from build123d import *

# Parameters (mm, degrees)
BOSS_EXTRUDE1_DEPTH = 0.43
SKETCH2_R           = 8.35
BOSS_EXTRUDE2_DEPTH = 1.7
CIRPATTERN1_COUNT   = 4
SKETCH3_R           = 7.25
BOSS_EXTRUDE3_DEPTH = 1.1
BOSS_EXTRUDE4_DEPTH = 3
FILLET1_R           = 0.4
FILLET2_R           = 1.5
FILLET3_R           = 6


with BuildPart() as part:
    # Sketch1 → Boss-Extrude1 (new body, symmetric)
    with BuildSketch(Plane.XY):
        Polygon((0, 0), (84.5, 0), (84.5, 6.75), (68.25, 6.75), (66.5, 4.25), (64.75, 6.75), (21.5, 6.75), (12.5, 4.5), (0, 4.5), align=None)
    boss_extrude1 = extrude(amount=BOSS_EXTRUDE1_DEPTH, both=True)

    # Sketch2 → Boss-Extrude2 (add)
    with BuildSketch(Plane.ZY):
        Circle(SKETCH2_R)
    extrude(amount=-BOSS_EXTRUDE2_DEPTH)

    # CirPattern1: Boss-Extrude1 ×4 about axis
    cirpattern1_axis = Axis((0, 0, 0), (1, 0, 0))
    for i in range(1, CIRPATTERN1_COUNT):
        add(boss_extrude1.rotate(cirpattern1_axis, i * 360 / CIRPATTERN1_COUNT))

    # Sketch3 → Boss-Extrude3 (add)
    with BuildSketch(Plane(origin=(84.5, 0, 0), x_dir=(0, 0, -1), z_dir=(1, 0, 0))):
        Circle(SKETCH3_R)
    extrude(amount=-BOSS_EXTRUDE3_DEPTH)

    # Sketch4 → Boss-Extrude4 (add)
    with BuildSketch(Plane(origin=(84.5, 0, 0), x_dir=(0, 0, -1), z_dir=(1, 0, 0))):
        Polygon((-3.8, -0.43), (-3.8, 0.43), (-0.43, 0.43), (-0.43, 3.8), (0.43, 3.8), (0.43, 0.43), (3.8, 0.43), (3.8, -0.43), (0.43, -0.43), (0.43, -3.8), (-0.43, -3.8), (-0.43, -0.43), align=None)
    extrude(amount=BOSS_EXTRUDE4_DEPTH)

    # Sketch6 → Revolve1 (revolve)
    with BuildSketch(Plane(origin=(0, 0, 0), x_dir=(1, 0, 0), z_dir=(0, 1, 0))):
        Polygon((87.5, 0), (88.3, 0), (88.3, -4.875), (87.5, -5.55), align=None)
    revolve(axis=Axis((87.5, 0, 0), (1, 0, 0)))

    # Fillet1
    fillet1_edges = [part.edges().sort_by_distance(p)[0] for p in [
        (66.5, 4.25, 0),
        (66.5, 0, 4.25),
        (66.5, -4.25, 0),
        (66.5, 0, -4.25),
    ]]
    fillet(fillet1_edges, radius=FILLET1_R)

    # Fillet2
    fillet2_edges = [part.edges().sort_by_distance(p)[0] for p in [
        (64.75, 6.75, 0),
        (68.25, 6.75, 0),
        (64.75, 0, 6.75),
        (68.25, 0, 6.75),
        (64.75, -6.75, 0),
        (68.25, -6.75, 0),
        (64.75, 0, -6.75),
        (68.25, 0, -6.75),
    ]]
    fillet(fillet2_edges, radius=FILLET2_R)

    # Fillet3
    fillet3_edges = [part.edges().sort_by_distance(p)[0] for p in [
        (12.5, 4.5, 0),
        (21.5, 6.75, 0),
        (12.5, 0, 4.5),
        (21.5, 0, 6.75),
        (12.5, -4.5, 0),
        (21.5, -6.75, 0),
        (12.5, 0, -4.5),
        (21.5, 0, -6.75),
    ]]
    fillet(fillet3_edges, radius=FILLET3_R)


solid = part.part
Geometry check sheet. Reference: the model listing, model coordinates, mm. A direction names the side the tool comes from. Round coordinates to 2 decimals unless told otherwise and drop trailing zeros. Loops run counter-clockwise (first coordinate to the right, second up) from the corner with the lowest first, then second, coordinate; pieces in that order, holes last. Notation, with made-up numbers: (20.25, -35) - (27.25, -35) arc R22 cw to (27.25, -10) - close; hole circle Ø10 at (-30.5, 79.25). An arc over 180 degrees is marked (long way). Answer as CSV lines item,"result".
(1) Cross-section at A-A, the plane x = 49. Enter the section's corners in (y, z).
Output values:
outline,"(-6.75, -0.43) - (-0.43, -0.43) - (-0.43, -6.75) - (0.43, -6.75) - (0.43, -0.43) - (6.75, -0.43) - (6.75, 0.43) - (0.43, 0.43) - (0.43, 6.75) - (-0.43, 6.75) - (-0.43, 0.43) - (-6.75, 0.43) - close"
(2) Set-up check for faces 4 (the face through (42, 4, -0.43)), 5 (the face through (83.96, -6.43, -3.35)), 6 (the face through (42, -4, -0.43)): record each of +Z, -Z, +X, -X, +Y, -Y from which the full face is reachable in a straight line by a thin tool's end or side.
Output values:
face 4,"-Z, +Y"
face 5,"+X"
face 6,"-Z, -Y"
(3) Release check for a two-part mould opening along X. For faces 1 (the face through (0.838, 2.508, 7.964)), 2 (the face through (88.3, 0, 0)), 3 (the face through (42, -4, 0.43)) record: released by +X, released by -X, zero draft, split by the parting line, or undercut.
Output values:
face 1,"zero draft"
face 2,"released by +X"
face 3,"undercut"
(4) Depth check by flat-ended pin: pin 1 Ø1.5 at (y, z) = (-5, 6.5) entering from +X; pin 2 Ø0.9 at (x, z) = (6.5, 0) entering from -Y; pin 3 Ø0.9 at (x, y) = (79, 0) entering from +Z. Enter the tip coordinate at first touch or a pass-through.
Output values:
pin 1,"stops at x = 1.7"
pin 2,"stops at y = -4.5"
pin 3,"stops at z = 6.75"
(5) Material ranges on line 1 along X through (y, z) = (-1.25, 2.25); line 2 along X through (y, z) = (-1.5, 4.75); line 3 along X through (y, z) = (6, 4), recorded low to high.
Output values:
line 1,"x = 0 to 1.7, 83.4 to 84.5, 87.5 to 88.3"
line 2,"x = 0 to 1.7, 83.4 to 84.5, 87.5 to 88.17"
line 3,"x = 0 to 1.7, 83.4 to 84.5"
